The listing builds one solid part. Answer for the finished solid, in the listing's coordinates (mm). A direction names the side the tool comes from. Round coordinates to 2 decimals unless told otherwise and drop trailing zeros. Loops run counter-clockwise (first coordinate to the right, second up) from the corner with the lowest first, then second, coordinate; pieces in that order, holes last. Notation, with made-up numbers: (-33.5, 61.5) - (-3.5, 61.5) arc R10 cw to (-3.5, 75.5) - close; hole circle Ø4 at (11.25, 4.25). An arc over 180 degrees is marked (long way). One line per question, with ' | ' between items. Start each with the question number.
from build123d import *

# Parameters (mm, degrees)
SKETCH1_W           = 12.7
SKETCH1_H           = 9.525
BOSS_EXTRUDE1_DEPTH = 2.54
FILLET1_R           = 0.635
SHELL1_START        = 0.635
SHELL1_OUTLINE_W    = 1.905
SHELL1_OUTLINE_H    = 8.255
SHELL1_DEPTH        = 11.43
SKETCH2_R           = 2.54
BOSS_EXTRUDE2_DEPTH = 1.905
BOSS_EXTRUDE3_DEPTH = 0.00254


# Read off the part's stored shape, not the designer's step: Shell1
with BuildPart() as part:
    # Sketch1 → Boss-Extrude1 (new body)
    with BuildSketch(Plane(origin=(0, 0, 0), x_dir=(1, 0, 0), z_dir=(0, 1, 0))):
        with Locations((6.35, 4.7625)):
            Rectangle(SKETCH1_W, SKETCH1_H)
    extrude(amount=BOSS_EXTRUDE1_DEPTH)

    # Fillet1
    fillet1_edges = [part.edges().sort_by_distance(p)[0] for p in [
        (0, 1.27, -9.525),
        (12.7, 1.27, -9.525),
        (12.7, 1.27, 0),
        (0, 1.27, 0),
    ]]
    fillet(fillet1_edges, radius=FILLET1_R)

    # Shell1 outline → Shell1 (cut)
    with BuildSketch(Plane.YZ.offset(SHELL1_START)):
        with Locations((0.9525, -4.7625)):
            Rectangle(SHELL1_OUTLINE_W, SHELL1_OUTLINE_H)
    extrude(amount=SHELL1_DEPTH, mode=Mode.SUBTRACT)

    # Sketch2 → Boss-Extrude2 (add)
    with BuildSketch(Plane(origin=(0, 1.905, 0), x_dir=(-1, 0, 0), z_dir=(0, -1, 0))):
        with Locations(Location((-6.35, 4.7625, 0), (0, 0, 270))):
            Circle(SKETCH2_R)
    extrude(amount=BOSS_EXTRUDE2_DEPTH)

    # Sketch3 → Boss-Extrude3 (add)
    with BuildSketch(Plane(origin=(0, 2.54, 0), x_dir=(1, 0, 0), z_dir=(0, 1, 0))):
        Polygon((4.557346154, 6.477), (6.104141026, 6.477), (6.104141026, 5.907128205), (5.127217949, 5.907128205), (5.127217949, 5.296551282), (6.104141026, 5.296551282), (6.104141026, 4.726679487), (5.127217949, 4.726679487), (5.127217949, 3.302), (4.557346154, 3.302), align=None)
        Polygon((6.551897436, 6.477), (8.587153846, 6.477), (8.587153846, 6.181251803), (7.186643029, 3.220589744), (6.681645032, 3.474996795), (7.851917468, 5.947833333), (6.551897436, 5.947833333), align=None)
    extrude(amount=BOSS_EXTRUDE3_DEPTH)


solid = part.part
(1) Find section B-B on z = -2. Write down the section's boundary in (x, y) (3 decimals).
(2) Consider L1, parallel to Z at x = 9.5, y = 1.6 (3 decimals); L2, parallel to Z at x = 7, y = 0.2 (3 decimals); L3, parallel to X at y = 1.3, z = -1 (3 decimals). Determine where each line is inside the solid, lowest interval first.
(3) Determine the mould class of faces 1 (the flat face through (5, 2.543, -5)), 2 (the flat face through (0.635, 1, -5)), 3 (the flat face through (0, 1, -5)) for opening direction X: pulls with the +X half, pulls with the -X half, needs draft (parallel to the pull), parting line crosses it, or undercut.
(4) Find section C-C on x = 6.35. Write down the section's boundary in (y, z) (1 decimal), plus the area to 3 significant figures.
(5) Find section D-D on x = 9.5. Write down the section's boundary in (y, z) (3 decimals).
(6) A tool of negligible diameter and unlimited length cuts with its end or side. For faces 4 (the cylindrical face through (8.603, 0.966, -3.59)), 5 (the flat face through (6, 1, -9.525)), from which of +Z, -Z, +X, -X, +Y, -Y can it reach the whole face along a straight path? Write none if from no direction.
(7) Find section A-A on y = 1.1. Count the separate pieces of the cut face and the enclosed holes in it, plus the area to 3 significant figures.
Answer below:
1) outline: (0, 0) - (0.635, 0) - (0.635, 1.905) - (12.065, 1.905) - (12.065, 0) - (12.7, 0) - (12.7, 2.54) - (0, 2.54) - close
2) L1: -9.525 to -8.89, -0.635 to 0 | L2: -9.525 to -8.89, -7.218 to -2.307, -0.635 to 0 | L3: 0 to 0.635, 12.065 to 12.7
3) face 1: needs draft | face 2: undercut | face 3: pulls with the -X half
4) outline: (0, -9.5) - (2.5, -9.5) - (2.5, 0) - (0, 0) - (0, -0.6) - (1.9, -0.6) - (1.9, -2.2) - (0, -2.2) - (0, -7.3) - (1.9, -7.3) - (1.9, -8.9) - (0, -8.9) - close | area: 18.1 mm2
5) outline: (0, -9.525) - (2.54, -9.525) - (2.54, 0) - (0, 0) - (0, -0.635) - (1.905, -0.635) - (1.905, -8.89) - (0, -8.89) - close
6) face 4: -Y | face 5: -Z, +X, -X, +Y, -Y
7) separate pieces: 2 | enclosed holes: 1 | area: 46.5 mm2
